The drawing under review shows one solid part. Ordinate dimensions are in mm from its lowest x, y, z. A direction names the side the tool comes from. Round coordinates to 2 decimals unless told otherwise and drop trailing zeros. Order: outer loops, then holes, each group sorted by start corner. A loop starts at its lowest first (then second) coordinate and runs counter-clockwise, first axis right, second up. Notation, with made-up numbers: (19, 44) -> (47, 44) arc R27 ccw to (47, 73) -> close; hole circle Ø8 at (-33, -4.75). An arc over 180 degrees is marked (long way). Use a Markdown table: item, result. Add a question column.
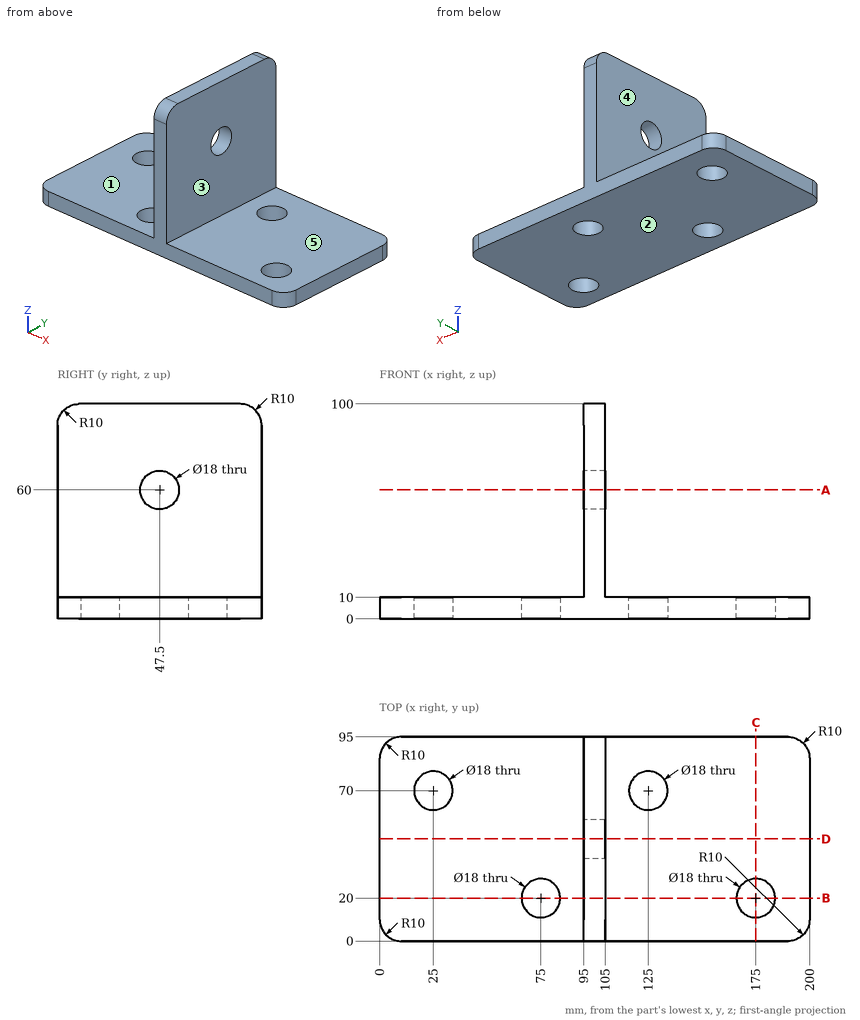
Q1. For pin 1 (16 mm diameter, centred on x = 125, y = 70, fed in from -Z); pin 2 (2 mm diameter, centred on x = 133, y = 33, fed in from +Z); pin 3 (8 mm diameter, centred on y = 70, z = 24, fed in from -X), all flat-tipped, find the tip position at first contact; note any pin that passes through.
Q2. Add section A-A, the plane z = 60. Give the boundary of the cut face in (x, y), then the cut area to 3 significant figures.
Q3. To check wall thickness, follow line 1 along X through (y, z) = (18, 6); line 2 along Z through (x, y) = (84.5, 23); line 3 along X through (y, z) = (63.5, 41). State the ranges of each line that lie inside material, in increasing order.
Q4. Draft analysis for pull direction X (two halves, no side actions). For the marked faces 3, 4 and 5, state which applies: released by +X, released by -X, zero draft, split by the parting line, or undercut.
Q5. Add section B-B, the plane y = 20. Give the boundary of the cut face in (x, z).
Q6. Add section C-C, the plane x = 175. Give the boundary of the cut face in (y, z).
Q7. Add section D-D, the plane y = 47.5. Give the boundary of the cut face in (x, z).
Q8. For the marked faces 1 and 2, list the 3-axis set-ups (+Z, -Z, +X, -X, +Y, -Y) from which the entire face can be reached by the end or side of a thin tool; tool diameter is ignored.
Return value:
| question | item | result |
|---|---|---|
| 1 | pin 1 | through |
| 1 | pin 2 | z = 10 |
| 1 | pin 3 | x = 95 |
| 2 | outline | (95, 0) -> (105, 0) -> (105, 38.5) -> (95, 38.5) -> close; (95, 56.5) -> (105, 56.5) -> (105, 95) -> (95, 95) -> close |
| 2 | area | 770 mm² |
| 3 | line 1 | 0 to 66.23, 83.77 to 166.23, 183.77 to 200 |
| 3 | line 2 | 0 to 10 |
| 3 | line 3 | 95 to 105 |
| 4 | face 3 | released by +X |
| 4 | face 4 | released by -X |
| 4 | face 5 | zero draft |
| 5 | outline | (0, 0) -> (66, 0) -> (66, 10) -> (0, 10) -> close; (84, 0) -> (166, 0) -> (166, 10) -> (105, 10) -> (105, 100) -> (95, 100) -> (95, 10) -> (84, 10) -> close; (184, 0) -> (200, 0) -> (200, 10) -> (184, 10) -> close |
| 6 | outline | (0, 0) -> (11, 0) -> (11, 10) -> (0, 10) -> close; (29, 0) -> (95, 0) -> (95, 10) -> (29, 10) -> close |
| 7 | outline | (0, 0) -> (200, 0) -> (200, 10) -> (105, 10) -> (105, 51) -> (95, 51) -> (95, 10) -> (0, 10) -> close; (95, 69) -> (105, 69) -> (105, 100) -> (95, 100) -> close |
| 8 | face 1 | +Z, -X, +Y, -Y |
| 8 | face 2 | -Z, +X, -X, +Y, -Y |
